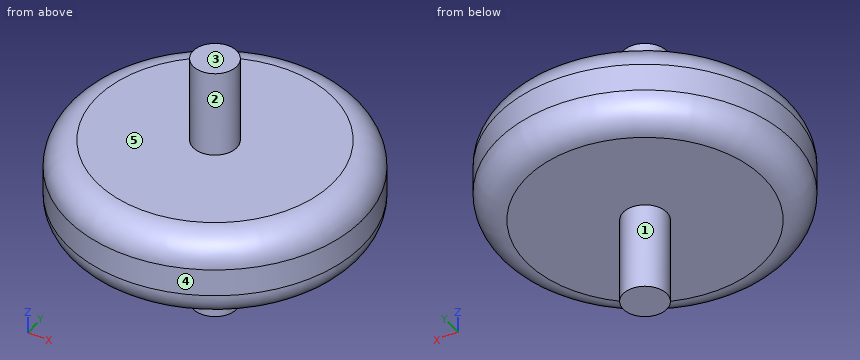
```python
from build123d import *

# Parameters (mm, degrees)
SKETCH1_R                = 101.6
BOSS_EXTRUDE1_DEPTH      = 59
FILLET1_R                = 20
SKETCH2_R                = 15
BOSS_EXTRUDE2_DEPTH      = 60
BOSS_EXTRUDE2_DEPTH_BACK = 119


with BuildPart() as part:
    # Sketch1 → Boss-Extrude1 (new body)
    with BuildSketch(Plane.XY):
        Circle(SKETCH1_R)
    extrude(amount=BOSS_EXTRUDE1_DEPTH)

    # Fillet1
    fillet1_edges = [part.edges().sort_by_distance(p)[0] for p in [
        (-101.6, 0, 0),
        (-101.6, 0, 59),
    ]]
    fillet(fillet1_edges, radius=FILLET1_R)

    # Sketch2 → Boss-Extrude2 (add, two sides)
    with BuildSketch(Plane.XY.offset(59)) as boss_extrude2_sk:
        Circle(SKETCH2_R)
    extrude(amount=BOSS_EXTRUDE2_DEPTH)
    extrude(boss_extrude2_sk.sketch, amount=-BOSS_EXTRUDE2_DEPTH_BACK)


solid = part.part
```
Here's how the part is built. I have some questions about the finished solid (model axes, mm). Face numbers are marked on the shaded views. A direction names the side the tool comes from. Coordinates: 2 decimals unless noted, no trailing zeros. Write each loop counter-clockwise with the first axis right and the second up, starting at its lowest first coordinate (ties: lowest second). Pieces come first, ordered by that corner, then holes. Notation, with made-up numbers: (55, 85.25) -> (114, 85.25) arc R9 ccw to (114, 91.25) -> close; hole circle Ø7 at (25.25, -23.75). An arc over 180 degrees is marked (long way). Use a Markdown table: item, result. Add a question column.
(1) For the marked faces 1, 2 and 3, which set-ups out of +Z, -Z, +X, -X, +Y, -Y let a thin tool reach every point of the face, with its end or its side?
(2) Please list where these lines run through material, in increasing order: line 1 (Z direction, x = -35, y = -29); line 2 (Y direction, x = -52, z = 31.5); line 3 (Z direction, x = 62.5, y = -72).
(3) If we section it at A-A, the plane x = 0: Write out the boundary of the cut face in (y, z), and give its area (3 significant figures).
(4) We'd pull the mould along Y, two halves only. Please class the marked faces 4 and 5: +Y half, -Y half, draft (parallel to the pull), parting line (faces both ways), or undercut.
(5) I'm going to push flat-ended pins straight in: P1, Ø2, axis at x = -9.5, z = 62.5, coming from the +Y side; P2, Ø2, axis at x = 26.5, y = 39.5, coming from the -Z side; P3, Ø5, axis at x = 0.5, z = 76, coming from the -Y side. Where does each tip first touch, or does it pass through?
(6) If we section it at D-D, the plane z = 8.5: Write out the boundary of the cut face in (x, y).
(7) If we section it at C-C, the plane z = 26.5: Write out the boundary of the cut face in (x, y).
Outcome:
| question | item | result |
|---|---|---|
| 1 | face 1 | -Z |
| 1 | face 2 | +Z |
| 1 | face 3 | +Z, +X, -X, +Y, -Y |
| 2 | line 1 | z = 0 to 59 |
| 2 | line 2 | y = -87.28 to 87.28 |
| 2 | line 3 | z = 5.47 to 53.53 |
| 3 | outline | (-101.6, 20) arc R20 ccw to (-81.6, 0) -> (-15, 0) -> (-15, -60) -> (15, -60) -> (15, 0) -> (81.6, 0) arc R20 ccw to (101.6, 20) -> (101.6, 39) arc R20 ccw to (81.6, 59) -> (15, 59) -> (15, 119) -> (-15, 119) -> (-15, 59) -> (-81.6, 59) arc R20 ccw to (-101.6, 39) -> close |
| 3 | area | 15,200 mm^2 |
| 4 | face 4 | parting line |
| 4 | face 5 | draft |
| 5 | P1 | stops at y = 12.36 |
| 5 | P2 | stops at z = 0 |
| 5 | P3 | stops at y = -15 |
| 6 | outline | circle Ø195.93 at (0, 0) |
| 7 | outline | circle Ø203.2 at (0, 0) |
